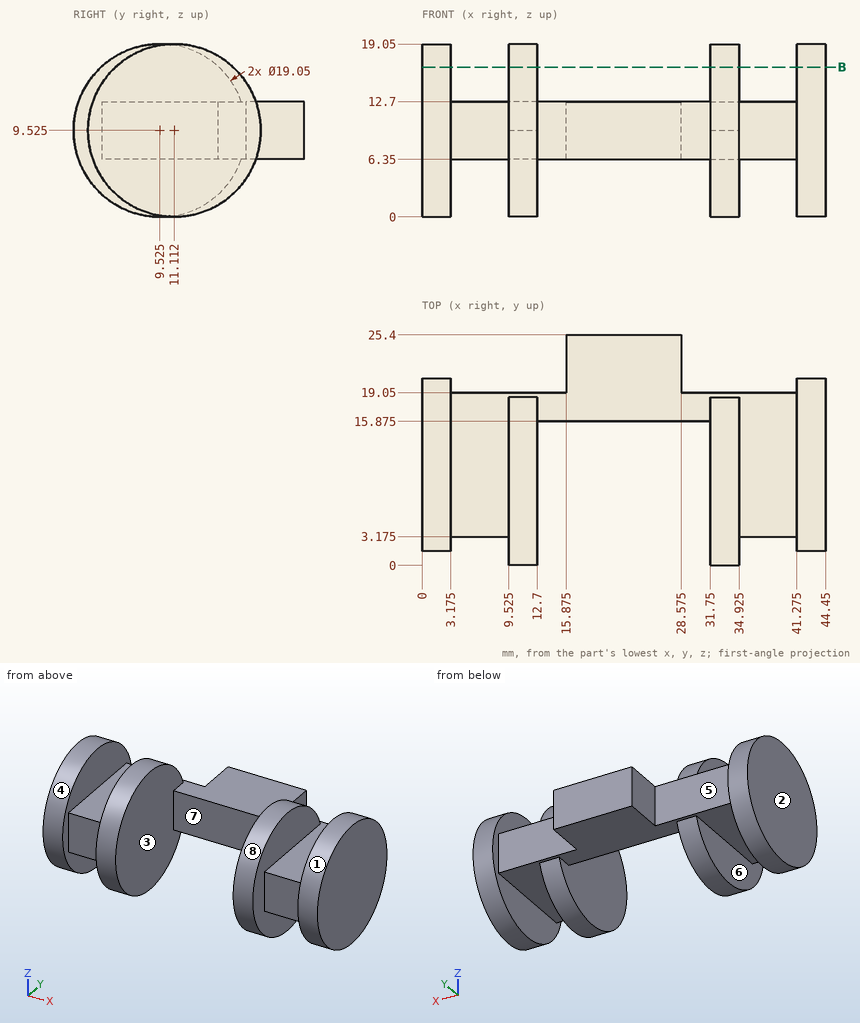
Could you check a few things on this drawing? It's one solid part, dimensions in mm from its lowest x, y, z. A direction names the side the tool comes from. Round coordinates to 2 decimals unless told otherwise and drop trailing zeros. One line per item, written item: value.
1) We'd pull the mould along X, two halves only. Please class the marked faces 1, 2 and 3: released by +X, released by -X, zero draft, split by the parting line, or undercut.
Filled sheet:
face 1: zero draft
face 2: released by -X
face 3: undercut
2) I'm going to push flat-ended pins straight in: pin 1 Ø3 at (x, z) = (35, 11) entering from +Y; pin 2 Ø1.5 at (y, z) = (21, 13) entering from -X (1 decimal); pin 3 Ø5 at (x, z) = (5, 11) entering from -Y. Where does each tip first touch, or does it pass through?
Filled sheet:
pin 1: stops at y = 19.05
pin 2: stops at x = 15.9
pin 3: stops at y = 1.59
3) For the marked faces 4, 5, 6, 7 and 8, which set-ups out of +Z, -Z, +X, -X, +Y, -Y let a thin tool reach every point of the face, with its end or its side?
Filled sheet:
face 4: -X
face 5: +Z, -Z, +Y
face 6: -Y
face 7: +Z, -Z, -Y
face 8: none
4) Suppose I cut it at B-B on z = 16.5. Give the number of separate pieces and of enclosed holes in the cut face, plus the area to 3 significant figures.
Filled sheet:
separate pieces: 4
enclosed holes: 0
area: 165 mm2
5) If I drill on line 1 (X direction, y = 3.25, z = 12); line 2 (X direction, y = 22.75, z = 9.75) (1 decimal); line 3 (Y direction, x = 42.5, z = 9.75) (1 decimal), over which ranges is the centre line in solid material (lowest first)? Write a range as [from, to].
Filled sheet:
line 1: x = [0, 12.7], [31.75, 44.45]
line 2: x = [15.9, 28.6]
line 3: y = [1.6, 20.6]
